Check sheet for the drawn part. Datum: minimum x, y, z corner. Units: mm. Give positions to 0.01 mm unless a question says otherwise; leave off trailing zeros. Write each loop counter-clockwise with the first axis right and the second up, starting at its lowest first coordinate (ties: lowest second). Pieces come first, ordered by that corner, then holes. Notation, with made-up numbers: (-31, 4) - (-23, 4) arc R8 cw to (-23, 17) - close; hole circle Ø1 at (-36, 85). An arc over 180 degrees is marked (long way). Use a Markdown table: item, result.
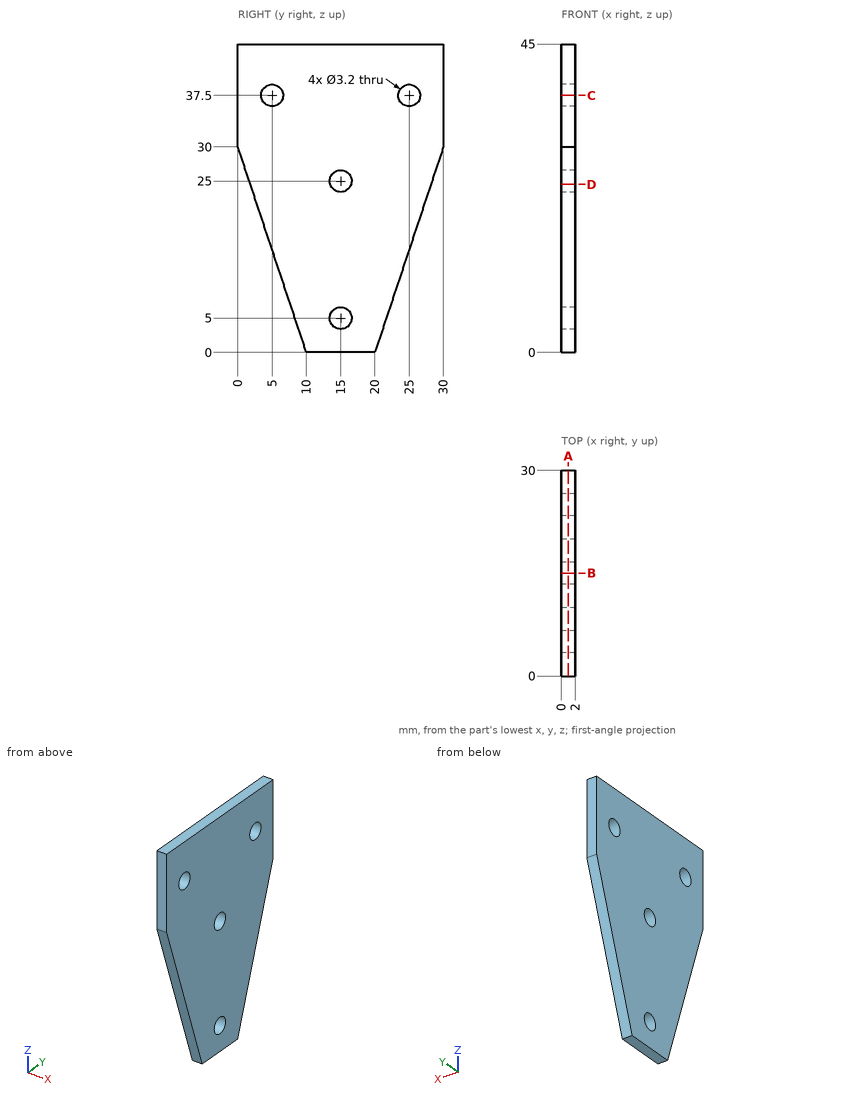
1) Depth check by flat-ended pin: P1, Ø2.5, axis at y = 25, z = 37.5, coming from the -X side. Enter the tip coordinate at first touch or a pass-through.
Working result:
| item | result |
|---|---|
| P1 | passes through |
2) Material ranges on L1, parallel to Y at x = 0.9, z = 37.5; L2, parallel to Y at x = 1.75, z = 6; L3, parallel to Y at x = 1.2, z = 25, recorded low to high. Write a range as from..to.
Working result:
| item | result |
|---|---|
| L1 | y = 0..3.4, 6.6..23.4, 26.6..30 |
| L2 | y = 8..13.75, 16.25..22 |
| L3 | y = 1.67..13.4, 16.6..28.33 |
3) Section check C-C on z = 37.5. Record the boundary of the cut face in (x, y).
Working result:
| item | result |
|---|---|
| outline | (0, 0) - (2, 0) - (2, 3.4) - (0, 3.4) - close; (0, 6.6) - (2, 6.6) - (2, 23.4) - (0, 23.4) - close; (0, 26.6) - (2, 26.6) - (2, 30) - (0, 30) - close |
4) Section check A-A on x = 1. Record the boundary of the cut face in (y, z).
Working result:
| item | result |
|---|---|
| outline | (0, 30) - (10, 0) - (20, 0) - (30, 30) - (30, 45) - (0, 45) - close; hole circle Ø3.2 at (5, 37.5); hole circle Ø3.2 at (15, 5); hole circle Ø3.2 at (15, 25); hole circle Ø3.2 at (25, 37.5) |
5) Section check D-D on z = 24.5. Record the boundary of the cut face in (x, y), then the cut area to 3 significant figures.
Working result:
| item | result |
|---|---|
| outline | (0, 1.83) - (2, 1.83) - (2, 13.48) - (0, 13.48) - close; (0, 16.52) - (2, 16.52) - (2, 28.17) - (0, 28.17) - close |
| area | 46.6 mm² |
6) Section check B-B on y = 15. Record the boundary of the cut face in (x, z), then the cut area to 3 significant figures.
Working result:
| item | result |
|---|---|
| outline | (0, 0) - (2, 0) - (2, 3.4) - (0, 3.4) - close; (0, 6.6) - (2, 6.6) - (2, 23.4) - (0, 23.4) - close; (0, 26.6) - (2, 26.6) - (2, 45) - (0, 45) - close |
| area | 77.2 mm² |
